The listing builds one solid part. Answer for the finished solid, in the listing's coordinates (mm). A direction names the side the tool comes from. Coordinates: 2 decimals unless noted, no trailing zeros. Order: outer loops, then holes, each group sorted by start corner. A loop starts at its lowest first (then second) coordinate and runs counter-clockwise, first axis right, second up. Notation, with made-up numbers: M 89.25,54 L 147.25,54 A21 ccw 147.25,62 Z; hole C 44,86.5 d2. An arc over 180 degrees is marked long. One line per item, written item: value. Start each with the question number.
Q1. Straight lines are drawn through the part: line 1 along X through (y, z) = (0, 1.4); line 2 along Y through (x, z) = (-10, 1.25); line 3 along X through (y, z) = (-1, 3.8). For each, find the intervals that lie inside material, in ascending order. Write a range as [from, to].
Q2. Determine the mould class of faces 1 (the flat face through (-10.737, -2.293, 2.712)), 2 (the flat face through (-9.21, 5.97, 2.71)), 3 (the flat face through (9, 9.3, 3)), 4 (the flat face through (-2.293, 10.737, 2.712)) for opening direction X: pulls with the +X half, pulls with the -X half, needs draft (parallel to the pull), parting line crosses it, or undercut.
Q3. Each of these flat-tipped pins is pushed along its axis until it touches: pin 1 Ø1 at (y, z) = (5.5, 4.5) entering from -X; pin 2 Ø3 at (x, z) = (-3.5, 1) entering from +Y; pin 3 Ø1.2 at (x, z) = (10, 3) entering from +Y. Where does it stop, or does it pass through?
Q4. The part is cut by section A-A on x = 0.75. Give the vertices of the cut face in (y, z), then the cut area to 3 significant figures.
Q5. For faces 5 (the flat face through (-7.381, -8.165, 2.712)), 6 (the flat face through (-10.993, -0.554, 2.712)), 7 (the flat face through (-4.994, 9.777, 2.712)), 8 (the flat face through (9, -10.7, 3)), 9 (the flat face through (-9.243, -5.977, 2.712)), determine the directions among +Z, -Z, +X, -X, +Y, -Y from which every point of the face is accessible in a straight line to the end or side of a thin tool.
```python
from build123d import *

# Parameters (mm, degrees)
SKETCH1_R           = 10
BOSS_EXTRUDE1_DEPTH = 5.5
BOSS_EXTRUDE2_DEPTH = 5.5
CIRPATTERN1_COUNT   = 24
SKETCH3_R           = 12.65
SKETCH3_R_2         = 12
CUT_EXTRUDE1_DEPTH  = 6
CUT_EXTRUDE2_DEPTH  = 6
SKETCH5_R           = 1.65
CUT_EXTRUDE3_DEPTH  = 6
BOSS_EXTRUDE3_DEPTH = 5.5


with BuildPart() as part:
    # Sketch1 → Boss-Extrude1 (new body)
    with BuildSketch(Plane.XY):
        Circle(SKETCH1_R)
    extrude(amount=BOSS_EXTRUDE1_DEPTH)

    # Sketch2 → Boss-Extrude2 (add)
    with BuildSketch(Plane.XY):
        with BuildLine():
            Line((0, 12.65), (-0.9, 9.959417654))
            ThreePointArc((-0.9, 9.959417654), (0, 10), (0.9, 9.959417654))
            Line((0.9, 9.959417654), (0, 12.65))
        make_face()
    boss_extrude2 = extrude(amount=BOSS_EXTRUDE2_DEPTH)

    # CirPattern1: Boss-Extrude2 ×24 about axis
    cirpattern1_axis = Axis((0, 0, 0), (0, 0, 1))
    for i in range(1, CIRPATTERN1_COUNT):
        add(boss_extrude2.rotate(cirpattern1_axis, i * 360 / CIRPATTERN1_COUNT))

    # Sketch3 → Cut-Extrude1 (cut)
    with BuildSketch(Plane.XY):
        Circle(SKETCH3_R)
        Circle(SKETCH3_R_2, mode=Mode.SUBTRACT)
    extrude(amount=CUT_EXTRUDE1_DEPTH, mode=Mode.SUBTRACT)

    # Sketch4 → Cut-Extrude2 (cut)
    with BuildSketch(Plane.XY):
        with BuildLine():
            Line((0, 0), (0, 12))
            ThreePointArc((0, 12), (11.769423365, -2.341083864), (-4.592201188, -11.08655439))
            Line((-4.592201188, -11.08655439), (-3.826834324, -9.238795325))
            Line((-3.826834324, -9.238795325), (0, 0))
        make_face()
    extrude(amount=CUT_EXTRUDE2_DEPTH, mode=Mode.SUBTRACT)

    # Sketch5 → Cut-Extrude3 (cut)
    with BuildSketch(Plane.XY):
        Circle(SKETCH5_R)
    extrude(amount=CUT_EXTRUDE3_DEPTH, mode=Mode.SUBTRACT)

    # Sketch6 → Boss-Extrude3 (add)
    with BuildSketch(Plane.XY):
        with BuildLine():
            Line((0, 1.65), (0, 12))
            Line((0, 12), (7, 12))
            Line((7, 12), (7, 9.3))
            Line((7, 9.3), (11, 9.3))
            Line((11, 9.3), (11, -10.7))
            Line((11, -10.7), (7, -10.7))
            Line((7, -10.7), (7, -14.3))
            Line((7, -14.3), (0, -14.3))
            Line((0, -14.3), (0, -10.7))
            Line((0, -10.7), (-3.826834324, -10.7))
            Line((-3.826834324, -10.7), (-3.826834324, -9.238795325))
            Line((-3.826834324, -9.238795325), (-0.631427663, -1.524401229))
            ThreePointArc((-0.631427663, -1.524401229), (1.618295713, -0.321899031), (0, 1.65))
        make_face()
    extrude(amount=BOSS_EXTRUDE3_DEPTH)


solid = part.part
```
Output:
1. line 1: x = [-12, -1.65], [1.65, 11]
1. line 2: y = [-6.13, -5.25], [-3.41, -1.81], [-0.89, 0.89], [1.81, 3.41], [5.25, 6.13]
1. line 3: x = [-9.95, -1.31], [1.31, 11]
2. face 1: pulls with the -X half
2. face 2: undercut
2. face 3: needs draft
2. face 4: undercut
3. pin 1: stops at x = -10.5
3. pin 2: stops at y = 11.65
3. pin 3: stops at y = 9.3
4. outline: M -14.3,0 L -1.47,0 L -1.47,5.5 L -14.3,5.5 Z; M 1.47,0 L 12,0 L 12,5.5 L 1.47,5.5 Z
4. area: 128 mm^2
5. face 5: +Z, -Z, -Y
5. face 6: +Z, -Z, -X
5. face 7: +Z, -Z, +Y
5. face 8: +Z, -Z, +X, -Y
5. face 9: +Z, -Z
